Read the model definition and answer for the solid it produces. Units are mm, in the model's axes. Round coordinates to 2 decimals unless told otherwise and drop trailing zeros. Order: outer loops, then holes, each group sorted by start corner. A loop starts at its lowest first (then second) coordinate and runs counter-clockwise, first axis right, second up. Notation, with made-up numbers: M 49.5,15.25 L 102.5,15.25 A23 ccw 102.5,34.25 Z; hole C -11,70.25 d7. An arc over 180 degrees is marked long. Answer as CSV lines item,"result".
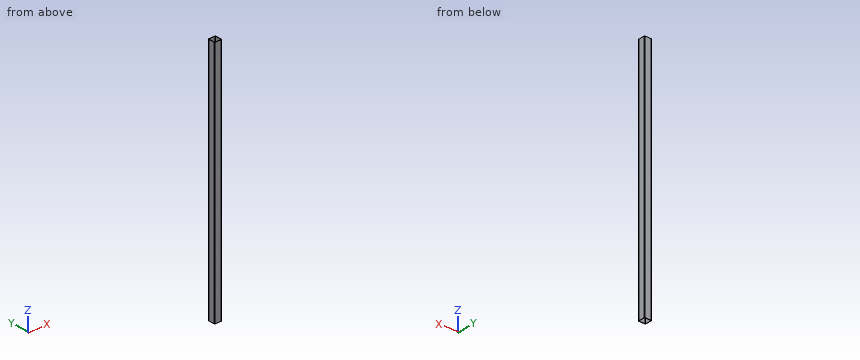
Autodesk Inventor part; units mm, degrees
ref_plane "Start Plane" through (0, 0, -25) normal (0, 0, 1) x (1, 0, 0)
ref_plane "End Plane" through (0, 0, 2335) normal (0, 0, 1) x (1, 0, 0)
ref_plane "Work Plane4" through (0, 21, -25) normal (0, 0, -1) x (-1, 0, 0)
ref_plane "Start Plane" through (0, 0, -25) normal (0, 0, 1) x (1, 0, 0)
ref_plane "End Plane" through (0, 0, 2335) normal (0, 0, 1) x (1, 0, 0)
sketch "Sketch" plane through (0, 0, 0) normal (0, 0, 1) x (1, 0, 0)
  line L0 (-35, -29) -> (-35, 29)
  line L1 (-29, 35) -> (29, 35)
  line L2 (35, 29) -> (35, -29)
  line L3 (29, -35) -> (-29, -35)
  arc A0 (-35, -29) -> (-29, -35) centre (-29, -29) ccw
  arc A1 (35, 29) -> (29, 35) centre (29, 29) ccw
  arc A2 (-29, 35) -> (-35, 29) centre (-29, 29) ccw
  arc A3 (29, -35) -> (35, -29) centre (29, -29) ccw
  arc A4 (-29, 32) -> (-32, 29) centre (-29, 29) ccw
  line L4 (-29, 32) -> (29, 32)
  arc A5 (32, 29) -> (29, 32) centre (29, 29) ccw
  line L5 (32, 29) -> (32, -29)
  arc A6 (29, -32) -> (32, -29) centre (29, -29) ccw
  line L6 (29, -32) -> (-29, -32)
  arc A7 (-32, -29) -> (-29, -32) centre (-29, -29) ccw
  line L7 (-32, -29) -> (-32, 29)
  line L8 (0, 50.7397) -> (0, -50.7397) construction
  line L9 (-50.7397, 0) -> (50.7397, 0) construction
  dimension "d7" = 6
  dimension "d9" = 70
  dimension "d11" = 70
  dimension "d12" = 3
  dimension "d15" = 35
  dimension "d16" = 35
extrude "Body" add sketch "Sketch" along normal up to surface (2360 mm away) from surface at -25
sketch "Sketch3" plane through (0, 0, 0) normal (0, 0, 1) x (1, 0, 0)
  line L0 (0, 0) -> (10, 0)
ref_plane "Work Plane3" through (0, 0, 0) normal (0, -1, 0) x (1, 0, 0)
sketch "Sketch4" plane through (0, 0, 0) normal (0, -1, 0) x (1, 0, 0)
  line L0 (-2, -25) -> (12, -25)
  line L1 (-2, 2335) -> (12, 2335)
  dimension "d18" = 2360
ref_plane "Work Plane4" through (0, 21, -25) normal (0, 0, -1) x (-1, 0, 0)
split "Split1" plane through (0, 21, -25) removes the side toward (0, 0, -1)
ref_plane "Work Plane5" through (0, -21, 2335) normal (0, 0, 1) x (1, 0, 0)
split "Split2" plane through (0, -21, 2335) removes the side toward (0, 0, 1)
equation "\"d7\" = G_IR"
equation "\"d9\" = G_W"
equation "\"d11\" = G_H"
equation "\"d12\" = G_T"
equation "\"d15\" = 0.5 * d9"
equation "\"d16\" = 0.5 * d11"
equation "\"d3\" = G_L"
equation "\"G_W\" = 70"
equation "\"G_H\" = 70"
equation "\"G_T\" = 3"
equation "\"G_IR\" = 6"
equation "\"G_L\" = d18"
equation "\"G_OFFSET_START\" = 25"
equation "\"G_OFFSET_END\" = 25"
equation "\"d13\" = -G_OFFSET_START"
equation "\"d14\" = G_OFFSET_END + B_L"
properties part number "ISO 10799-2 - 70x70x3 - 2360" material "Galvanizado catalogo 2"
Item 1: A cutting plane is placed at B-B, the plane x = -17. Determine the outline of the cut face in (y, z), and give its area (3 significant figures).
Ans:
outline,"M -35,-25 L -32,-25 L -32,2335 L -35,2335 Z; M 32,-25 L 35,-25 L 35,2335 L 32,2335 Z"
area,"14,200 mm2"
Item 2: Find the intervals of material crossed by probe 1 along X at (y, z) = (7, 1085), in increasing order. Write a range as [from, to].
Ans:
probe 1,"[-35, -32], [32, 35]"
Item 3: A cutting plane is placed at A-A, the plane z = 654. Determine the outline of the cut face in (x, y), and give its area (3 significant figures).
Ans:
outline,"M -35,-29 A6 ccw -29,-35 L 29,-35 A6 ccw 35,-29 L 35,29 A6 ccw 29,35 L -29,35 A6 ccw -35,29 Z; hole M -32,-29 A3 ccw -29,-32 L 29,-32 A3 ccw 32,-29 L 32,29 A3 ccw 29,32 L -29,32 A3 ccw -32,29 Z"
area,"781 mm2"
